```python
from build123d import *

# Parameters (mm, degrees)
F0_R     = 10.668
F0_R_2   = 7.747
F1_DEPTH = 95.25
F2_R     = 15.24
F2_R_2   = 10.668
F2_R_3   = 7.747
F3_DEPTH = 6.35
F4_R     = 10.668
F4_R_2   = 7.747
F5_DEPTH = 127
F6_R     = 3.175
F7_DEPTH = 12.7
F8_R     = 5.08
F9_DEPTH = 25.4


with BuildPart() as f1:
    # F0 (on Top) → F1 (new body)
    with BuildSketch(Plane.XY):
        Circle(F0_R)
        Circle(F0_R_2, mode=Mode.SUBTRACT)
    extrude(amount=F1_DEPTH)

    # F2 (on face) → F3 (join)
    with BuildSketch(Plane.XY.offset(95.25)):
        Circle(F2_R)
        Circle(F2_R_2, mode=Mode.SUBTRACT)
        Circle(F2_R_2)
        Circle(F2_R_3, mode=Mode.SUBTRACT)
    extrude(amount=F3_DEPTH)

    # F4 (on face) → F5 (join)
    with BuildSketch(Plane.XY.offset(101.6)):
        Circle(F4_R)
        Circle(F4_R_2, mode=Mode.SUBTRACT)
    extrude(amount=F5_DEPTH)

    # F6 (on Right) → F7 (cut, symmetric)
    with BuildSketch(Plane.YZ):
        with Locations((0, 203.2)):
            Circle(F6_R)
    extrude(amount=F7_DEPTH, both=True, mode=Mode.SUBTRACT)

    # F8 (on Front) → F9 (cut)
    with BuildSketch(Plane.XZ):
        with Locations((0, 114.3)):
            Circle(F8_R)
        with Locations((0, 158.75)):
            Circle(F8_R)
        with Locations((0, 203.2)):
            Circle(F8_R)
    extrude(amount=-F9_DEPTH, mode=Mode.SUBTRACT)


solid = f1.part
```
For this review, take the finished solid that the model builds, in its own axes (mm). A direction names the side the tool comes from. Coordinates: 2 decimals unless noted, no trailing zeros. Loops run counter-clockwise (first coordinate to the right, second up) from the corner with the lowest first, then second, coordinate; pieces in that order, holes last. Notation, with made-up numbers: (66, 27.5) -> (93, 27.5) arc R31 cw to (93, 58.5) -> close; hole circle Ø7 at (44.25, -32). An arc over 180 degrees is marked (long way). Return JSON: item names as keys, results as strings. Group by question number.
(1) Consider section D-D, the plane z = 114.3. Give the boundary of the cut face in (x, y), plus the area to 3 significant figures.
(2) Consider section B-B, the plane y = 0. Give the boundary of the cut face in (x, z) (3 decimals).
(3) Tool access review of faces 1 (the flat face through (-10.4, -3.2, 101.6)), 2 (the cylindrical face through (4.923, -9.464, 46.958)), 3 (the cylindrical face through (-8.85, 3.03, 204.15)), 4 (the cylindrical face through (-1.1, 8.22, 109.34)), 5 (the cylindrical face through (-1.679, -7.563, 112.7)): name each direction out of +Z, -Z, +X, -X, +Y, -Y from which nothing blocks a thin tool from reaching the whole face with its end or side.
(4) Mouldability with a two-part tool opening along Y and no side actions: class faces 6 (the cylindrical face through (8.89, 3.03, 204.15)), 7 (the cylindrical face through (-2.313, -10.414, 164.211)), 8 (the flat face through (-6, 6, 0)) as pulls with the +Y half, pulls with the -Y half, needs draft (parallel to the pull), parting line crosses it, or undercut.
(5) Consider section C-C, the plane z = 203.2. Give the boundary of the cut face in (x, y) (1 decimal).
(6) To check wall thickness, follow L1, parallel to Z at x = 0, y = 8.7; L2, parallel to X at y = 8, z = 203.2; L3, parallel to X at y = 0, z = 118. State the ranges of each line that lie inside material, in increasing order.
(7) Consider section A-A, the plane x = 0. Give the boundary of the cut face in (y, z).
(8) For pin 1 Ø12 at (x, z) = (-9.5, 132.5) entering from +Y; pin 2 Ø3 at (x, z) = (7.5, 95) entering from -Y; pin 3 Ø1.5 at (x, y) = (6.5, -2.5) entering from +Z; pin 4 Ø13 at (x, z) = (0, 114.3) entering from +Y, all flat-tipped, find the tip position at first contact; note any pin that passes through.
Results below:
{
 "1": {"outline": "(-5.08, 5.85) -> (-5.08, 9.38) arc R10.67 ccw (long way) to (5.08, 9.38) -> (5.08, 5.85) arc R7.75 cw (long way) to start", "area": "137 mm2"},
 "2": {"outline": "(-15.24, 95.25) -> (-10.668, 95.25) -> (-10.668, 0) -> (-7.747, 0) -> (-7.747, 200.025) -> (-10.668, 200.025) -> (-10.668, 101.6) -> (-15.24, 101.6) -> close; (-10.668, 206.375) -> (-7.747, 206.375) -> (-7.747, 228.6) -> (-10.668, 228.6) -> close; (7.747, 0) -> (10.668, 0) -> (10.668, 95.25) -> (15.24, 95.25) -> (15.24, 101.6) -> (10.668, 101.6) -> (10.668, 200.025) -> (7.747, 200.025) -> close; (7.747, 206.375) -> (10.668, 206.375) -> (10.668, 228.6) -> (7.747, 228.6) -> close"},
 "3": {"face 1": "+Z", "face 2": "-Z", "face 3": "+X, -X", "face 4": "+Y", "face 5": "+Z, -Z"},
 "4": {"face 6": "undercut", "face 7": "parting line crosses it", "face 8": "needs draft"},
 "5": {"outline": "(-10.2, -3.2) arc R10.7 ccw to (10.2, -3.2) -> (7.1, -3.2) arc R7.7 cw to (-7.1, -3.2) -> close; (-10.2, 3.2) -> (-7.1, 3.2) arc R7.7 cw to (-5.1, 5.8) -> (-5.1, 9.4) arc R10.7 ccw to start; (5.1, 5.8) arc R7.7 cw to (7.1, 3.2) -> (10.2, 3.2) arc R10.7 ccw to (5.1, 9.4) -> close"},
 "6": {"L1": "z = 0 to 109.22, 119.38 to 153.67, 163.83 to 198.12, 208.28 to 228.6", "L2": "x = -7.06 to -5.08, 5.08 to 7.06", "L3": "x = -10.67 to -7.75, 7.75 to 10.67"},
 "7": {"outline": "(-15.24, 95.25) -> (-10.67, 95.25) -> (-10.67, 0) -> (-7.75, 0) -> (-7.75, 228.6) -> (-10.67, 228.6) -> (-10.67, 101.6) -> (-15.24, 101.6) -> close; (7.75, 0) -> (10.67, 0) -> (10.67, 95.25) -> (15.24, 95.25) -> (15.24, 101.6) -> (10.67, 101.6) -> (10.67, 109.22) -> (7.75, 109.22) -> close; (7.75, 119.38) -> (10.67, 119.38) -> (10.67, 153.67) -> (7.75, 153.67) -> close; (7.75, 163.83) -> (10.67, 163.83) -> (10.67, 198.12) -> (7.75, 198.12) -> close; (7.75, 208.28) -> (10.67, 208.28) -> (10.67, 228.6) -> (7.75, 228.6) -> close"},
 "8": {"pin 1": "stops at y = 10.08", "pin 2": "stops at y = -14", "pin 3": "passes through", "pin 4": "stops at y = 10.67"}
}
